Design review of the part built by this model. Coordinates are the model's own, in mm. A direction names the side the tool comes from. Give positions to 0.01 mm unless a question says otherwise; leave off trailing zeros. Order: outer loops, then holes, each group sorted by start corner. A loop starts at its lowest first (then second) coordinate and runs counter-clockwise, first axis right, second up. Notation, with made-up numbers: (-14, 84.5) -> (36, 84.5) arc R10 ccw to (36, 98.5) -> close; hole circle Ø3 at (-19, -38.5). An arc over 180 degrees is marked (long way). One line per item, written item: value. Start each with the question number.
1) For pin 1 (1.5 mm diameter, centred on y = 36.5, z = 17, fed in from -X), flat-tipped, find the tip position at first contact; note if it passes through.
2) The part is to be moulded in two halves that separate along Y. For faces 1 (the face through (-1, 112.732, 17)), 2 (the face through (-37.5, 3, 17)), 3 (the face through (-36, 22.732, 17)), say which applies: released by +Y, released by -Y, zero draft, split by the parting line, or undercut.
3) Consider section B-B (y = 71). State the section outline as (x, z) points.
4) Consider section A-A (z = 16.7). State the section outline as (x, y) points.
5) Tool access review of faces 4 (the face through (-36, 82.732, 17)), 5 (the face through (-37.5, 53, 17)): name each direction out of +Z, -Z, +X, -X, +Y, -Y from which nothing blocks a thin tool from reaching the whole face with its end or side.
6) Wall thickness on line 1 along X through (y, z) = (68, 18.25): over which ranges is the line inside the solid? List them lowest first. Write a range as from..to.
from build123d import *

# Parameters (mm, degrees)
F0_W     = 5.3952559829
F0_H     = 21.7885393649
F0_W_2   = 6.4328089356
F0_H_2   = 60.9454013749
F1_DEPTH = 12.5
F3_W     = 25
F3_H     = 62.590439771
F4_DEPTH = 146.2136954069
F5_DEPTH = 25
F6_W     = 3
F6_H     = 15
F6_W_2   = 50
F6_H_2   = 1.2136954069
F7_DEPTH = 3
F8_DEPTH = 25


with BuildPart() as f1:
    # F0 (on Right) → F1 (new body, symmetric)
    with BuildSketch(Plane.YZ):
        with Locations((-29.570158571, 3.008893691)):
            Rectangle(F0_W, F0_H)
        Polygon((113.9459088445, 18.5482017696), (-32.2677865624, 18.5482017696), (-32.2677865624, 13.9031633735), (-26.8725305796, 13.9031633735), (107.5130999088, 13.9031633735), (113.9459088445, 13.9031633735), align=None)
        with Locations((110.7295043766, -16.569537314)):
            Rectangle(F0_W_2, F0_H_2)
    extrude(amount=F1_DEPTH, both=True)

    # F3 (on face) → F4 (cut, through all)
    with BuildSketch(Plane(origin=(0, 113.9459088445, 0), x_dir=(-1, 0, 0), z_dir=(0, 1, 0))):
        with Locations((0, -15.7470181159)):
            Rectangle(F3_W, F3_H)
    extrude(amount=-F4_DEPTH, mode=Mode.SUBTRACT)

    # F5 (add): a face of the model
    f5_faces = [f1.faces().sort_by_distance(p)[0] for p in [
        (-12.5, 40.839061141, 17.0482017696),
    ]]
    extrude(f5_faces, amount=F5_DEPTH)

    # F6 (on face) → F7 (cut, through all)
    with BuildSketch(Plane.XY.offset(18.5482017696)):
        with Locations((-36, -9.7677865624)):
            Rectangle(F6_W, F6_H)
        with Locations((-36, 15.2322134376)):
            Rectangle(F6_W, F6_H)
        with Locations((-36, 40.2322134376)):
            Rectangle(F6_W, F6_H)
        with Locations((-36, 65.2322134376)):
            Rectangle(F6_W, F6_H)
        with Locations((-36, 90.2322134376)):
            Rectangle(F6_W, F6_H)
        with Locations((-12.5, 113.339061141)):
            Rectangle(F6_W_2, F6_H_2)
    extrude(amount=-F7_DEPTH, mode=Mode.SUBTRACT)

    # F8 (add): a face of the model
    f8_faces = [f1.faces().sort_by_distance(p)[0] for p in [
        (12.5, 40.2322134376, 17.0482017696),
    ]]
    extrude(f8_faces, amount=F8_DEPTH)


solid = f1.part
Checked values:
1. pin 1: stops at x = -34.5
2. face 1: released by +Y
2. face 2: zero draft
2. face 3: undercut
3. outline: (-34.5, 15.55) -> (37.5, 15.55) -> (37.5, 18.55) -> (-34.5, 18.55) -> close
4. outline: (-37.5, -32.27) -> (37.5, -32.27) -> (37.5, 112.73) -> (-37.5, 112.73) -> (-37.5, 97.73) -> (-34.5, 97.73) -> (-34.5, 82.73) -> (-37.5, 82.73) -> (-37.5, 72.73) -> (-34.5, 72.73) -> (-34.5, 57.73) -> (-37.5, 57.73) -> (-37.5, 47.73) -> (-34.5, 47.73) -> (-34.5, 32.73) -> (-37.5, 32.73) -> (-37.5, 22.73) -> (-34.5, 22.73) -> (-34.5, 7.73) -> (-37.5, 7.73) -> (-37.5, -2.27) -> (-34.5, -2.27) -> (-34.5, -17.27) -> (-37.5, -17.27) -> close
5. face 4: +Z, -Z, -X
5. face 5: +Z, -Z, -X, +Y, -Y
6. line 1: x = -34.5..37.5
